```python
from build123d import *

# Parameters (mm, degrees)
SKETCH1_R           = 17.35
BOSS_EXTRUDE1_DEPTH = 60
SKETCH2_R           = 18.9
BOSS_EXTRUDE2_DEPTH = 37
BOSS_EXTRUDE4_DEPTH = 3
BOSS_EXTRUDE3_DEPTH = 21.3


with BuildPart() as part:
    # Sketch1 → Boss-Extrude1 (new body)
    with BuildSketch(Plane.XY):
        Circle(SKETCH1_R)
    extrude(amount=BOSS_EXTRUDE1_DEPTH)

    # Sketch2 → Boss-Extrude2 (add)
    with BuildSketch(Plane.XY.offset(60)):
        Circle(SKETCH2_R)
    extrude(amount=BOSS_EXTRUDE2_DEPTH)

    # Sketch4 → Boss-Extrude4 (add)
    with BuildSketch(Plane.XY.offset(97)):
        with BuildLine():
            Line((20, 21.1), (20, -21.1))
            Line((20, -21.1), (-20, -21.1))
            Line((-20, -21.1), (-20, 21.1))
            Line((-20, 21.1), (-20, 30))
            Line((-20, 30), (-18, 30))
            Line((-18, 30), (-18, 27.4))
            ThreePointArc((-18, 27.4), (-15.3, 24.7), (-12.6, 27.4))
            Line((-12.6, 27.4), (-12.6, 30))
            Line((-12.6, 30), (12.6, 30))
            Line((12.6, 30), (12.6, 27.4))
            ThreePointArc((12.6, 27.4), (15.3, 24.7), (18, 27.4))
            Line((18, 27.4), (18, 30))
            Line((18, 30), (20, 30))
            Line((20, 30), (20, 21.1))
        make_face()
    extrude(amount=BOSS_EXTRUDE4_DEPTH)

    # Sketch3 → Boss-Extrude3 (add)
    with BuildSketch(Plane.XY.offset(97)):
        with BuildLine():
            Line((1.5, 3.6), (0, 3.6))
            Line((0, 3.6), (-1.5, 3.6))
            ThreePointArc((-1.5, 3.6), (0, -3.9), (1.5, 3.6))
        make_face()
    extrude(amount=BOSS_EXTRUDE3_DEPTH)


solid = part.part
```
Model file for the job. Use its own axes, mm. A direction names the side the tool comes from. Give positions to 0.01 mm unless a question says otherwise; leave off trailing zeros. Write each loop counter-clockwise with the first axis right and the second up, starting at its lowest first coordinate (ties: lowest second). Pieces come first, ordered by that corner, then holes. Notation, with made-up numbers: (71.25, 63) -> (80.25, 63) arc R16 ccw to (80.25, 70) -> close; hole circle Ø4 at (27, 66). An arc over 180 degrees is marked (long way). Use CSV: the item, a comma, the result in double quotes. Start each with the question number.
1) Tool access for faces 1 (the flat face through (0, 3.6, 109)), 2 (the cylindrical face through (-0.1, -3.9, 109)), 3 (the flat face through (-20, 4, 98)), 4 (the flat face through (-12.6, 29, 98)), 5 (the cylindrical face through (-2.259, 17.202, 29.58)): list every direction of +Z, -Z, +X, -X, +Y, -Y with a clear straight run to the whole face (end or side of a thin tool).
2) Cut at A-A on y = 0. List the corners of the cut face in (x, z), plus the area to 3 significant figures.
3) Drill centre lines: L1, parallel to Z at x = 10, y = 8; L2, parallel to Z at x = 1, y = 25; L3, parallel to X at y = -7.5, z = 70. Where is each one in solid material? Low to high.
4) Two-plate mould, pull along X, no slides. Class faces 6 (the cylindrical face through (-15.4, 24.7, 98.5)), 7 (the flat face through (0, 5, 100)), 8 (the flat face through (20, 5, 98)): released by +X, released by -X, zero draft, split by the parting line, or undercut.
5) Cut at C-C on z = 82. List the corners of the cut face in (x, y), plus the area to 3 significant figures.
6) Pin check, flat tips, straight feed: P1, Ø2.5, axis at x = 0, z = 105.5, coming from the +Y side; P2, Ø12, axis at x = -2, z = 29.5, coming from the -Y side; P3, Ø1, axis at y = 4.5, z = 48.5, coming from the +X side. Stop position of each tip, or through.
7) Cut at D-D on x = -15.3. List the corners of the cut face in (y, z), plus the area to 3 significant figures.
8) Cut at B-B on x = 0. List the corners of the cut face in (y, z).
Final values:
1,face 1,"+Z, +X, -X, +Y"
1,face 2,"+Z"
1,face 3,"+Z, -Z, -X, +Y, -Y"
1,face 4,"+Z, -Z, +Y"
1,face 5,"-Z"
2,outline,"(-20, 97) -> (-18.9, 97) -> (-18.9, 60) -> (-17.35, 60) -> (-17.35, 0) -> (17.35, 0) -> (17.35, 60) -> (18.9, 60) -> (18.9, 97) -> (20, 97) -> (20, 100) -> (3.9, 100) -> (3.9, 118.3) -> (-3.9, 118.3) -> (-3.9, 100) -> (-20, 100) -> close"
2,area,"3,740 mm2"
3,L1,"z = 0 to 100"
3,L2,"z = 97 to 100"
3,L3,"x = -17.35 to 17.35"
4,face 6,"undercut"
4,face 7,"zero draft"
4,face 8,"released by +X"
5,outline,"circle Ø37.8 at (0, 0)"
5,area,"1,120 mm2"
6,P1,"stops at y = 3.6"
6,P2,"stops at y = -17.35"
6,P3,"stops at x = 16.88"
7,outline,"(-21.1, 97) -> (-11.1, 97) -> (-11.1, 60) -> (-8.18, 60) -> (-8.18, 0) -> (8.18, 0) -> (8.18, 60) -> (11.1, 60) -> (11.1, 97) -> (24.7, 97) -> (24.7, 100) -> (-21.1, 100) -> close"
7,area,"1,940 mm2"
8,outline,"(-21.1, 97) -> (-18.9, 97) -> (-18.9, 60) -> (-17.35, 60) -> (-17.35, 0) -> (17.35, 0) -> (17.35, 60) -> (18.9, 60) -> (18.9, 97) -> (30, 97) -> (30, 100) -> (3.6, 100) -> (3.6, 118.3) -> (-3.9, 118.3) -> (-3.9, 100) -> (-21.1, 100) -> close"
